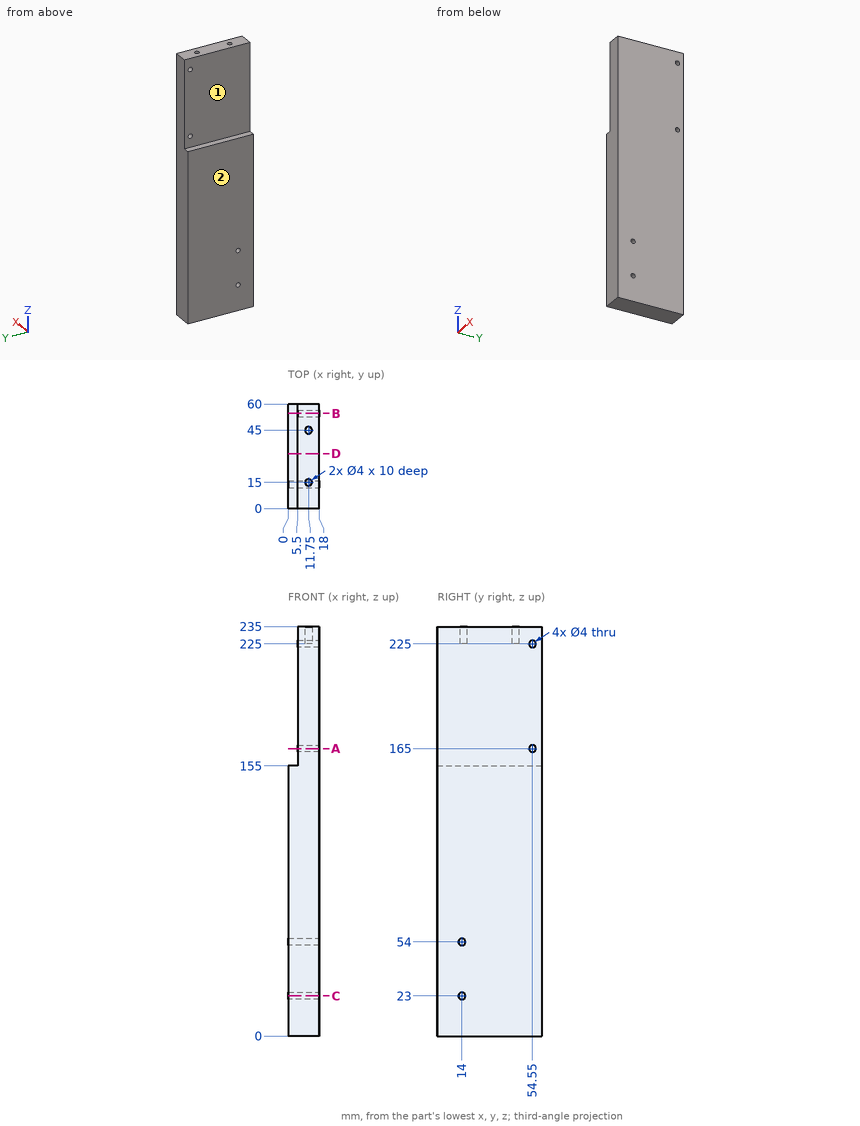
Geometry: see drawing. Coordinates: mm, zero at the bounding-box minimum. A direction names the side the tool comes from. Give positions to 0.01 mm unless a question says otherwise; leave off trailing zeros. Order: outer loops, then holes, each group sorted by start corner. A loop starts at its lowest first (then second) coordinate and runs counter-clockwise, first axis right, second up. Notation, with made-up numbers: (6, -11.5) -> (62, -11.5) arc R20 ccw to (62, 27.5) -> close; hole circle Ø6 at (29.5, 71). An arc over 180 degrees is marked (long way). Write each question's results on one line, items separated by ' | '.
1) Cut plane D-D (y = 31.5). Output: boundary loops of the cut face in (x, z), and give its area (3 significant figures).
Geometry says:
outline: (0, 0) -> (18, 0) -> (18, 235) -> (5.5, 235) -> (5.5, 155) -> (0, 155) -> close | area: 3,790 mm²
2) First-contact query: pin 1 Ø4 at (y, z) = (41.5, 186) entering from -X; pin 2 Ø1.6 at (x, y) = (1.5, 29.5) entering from +Z; pin 3 Ø3.5 at (x, y) = (11.75, 45) entering from +Z; pin 4 Ø3 at (y, z) = (14, 54) entering from +X. Flat tips, straight axial feed; report the tip coordinate or a pass-through.
Geometry says:
pin 1: stops at x = 5.5 | pin 2: stops at z = 155 | pin 3: stops at z = 225 | pin 4: passes through
3) Cut plane B-B (y = 54.55). Output: boundary loops of the cut face in (x, z), and give its area (3 significant figures).
Geometry says:
outline: (0, 0) -> (18, 0) -> (18, 163) -> (5.5, 163) -> (5.5, 155) -> (0, 155) -> close; (5.5, 167) -> (18, 167) -> (18, 223) -> (5.5, 223) -> close; (5.5, 227) -> (18, 227) -> (18, 235) -> (5.5, 235) -> close | area: 3,690 mm²
4) Cut plane C-C (z = 23). Output: boundary loops of the cut face in (x, y), and give its area (3 significant figures).
Geometry says:
outline: (0, 0) -> (18, 0) -> (18, 12) -> (0, 12) -> close; (0, 16) -> (18, 16) -> (18, 60) -> (0, 60) -> close | area: 1,010 mm²
5) Line query: line 1 along Y through (x, z) = (11.75, 229.5); line 2 along Y through (x, z) = (9, 225); line 3 along Z through (x, y) = (8.5, 15.5). Output: solid intervals per line, ascending.
Geometry says:
line 1: y = 0 to 13, 17 to 43, 47 to 60 | line 2: y = 0 to 52.55, 56.55 to 60 | line 3: z = 0 to 21.68, 24.32 to 52.68, 55.32 to 235
6) Cut plane A-A (z = 165). Output: boundary loops of the cut face in (x, y), and give its area (3 significant figures).
Geometry says:
outline: (5.5, 0) -> (18, 0) -> (18, 52.55) -> (5.5, 52.55) -> close; (5.5, 56.55) -> (18, 56.55) -> (18, 60) -> (5.5, 60) -> close | area: 700 mm²
7) Set-up query: the marked faces 1 and 2. Return all of +Z, -Z, +X, -X, +Y, -Y with unobstructed straight access to the full face (end or side cutting, diameter ignored); none if empty.
Geometry says:
face 1: +Z, -X, +Y, -Y | face 2: +Z, -Z, -X, +Y, -Y
